```python
from build123d import *

# Parameters (mm, degrees)
ESQUISSE1_W                                  = 200
ESQUISSE1_H                                  = 160
ESQUISSE1_R                                  = 5
ESQUISSE1_R_2                                = 1.75
ESQUISSE1_W_2                                = 10
ESQUISSE1_H_2                                = 10
ESQUISSE1_H_3                                = 30
BOSS_EXTRU_1_DEPTH                           = 5
CONG_2_R                                     = 1
ENL_V_MAT_EXTRU_1_DEPTH                      = 129.16005618
ESQUISSE3_R                                  = 1.75
TROU_CUVE_DIRECTION_DEPTH                    = 129.16005618
ESQUISSE4_R                                  = 1.7
ESQUISSE4_R_2                                = 5
POINTE_AVANT_TROUS_BATTERIES_ET_CABLES_DEPTH = 129.16005618


with BuildPart() as part:
    # Esquisse1 → Boss.-Extru.1 (new body)
    with BuildSketch(Plane(origin=(0, 0, 0), x_dir=(0, 1, 0), z_dir=(0, 0, 1))):
        Rectangle(ESQUISSE1_W, ESQUISSE1_H)
        with Locations(Location((-75, 0, 0), (0, 0, 270))):
            Circle(ESQUISSE1_R, mode=Mode.SUBTRACT)
        with Locations(Location((-57.5, 35.5, 0), (0, 0, 270))):
            Circle(ESQUISSE1_R_2, mode=Mode.SUBTRACT)
        with Locations(Location((-57.5, -35.5, 0), (0, 0, 90))):
            Circle(ESQUISSE1_R_2, mode=Mode.SUBTRACT)
        with Locations(Location((65, 45, 0), (0, 0, 270))):
            Circle(ESQUISSE1_R_2, mode=Mode.SUBTRACT)
        with Locations(Location((65, -45, 0), (0, 0, 90))):
            Circle(ESQUISSE1_R_2, mode=Mode.SUBTRACT)
        with Locations(Location((-31, 37.5, 0), (0, 0, 270))):
            Circle(ESQUISSE1_R_2, mode=Mode.SUBTRACT)
        with Locations(Location((-31, 75, 0), (0, 0, 270))):
            Circle(ESQUISSE1_R_2, mode=Mode.SUBTRACT)
        with Locations(Location((6.5, 75, 0), (0, 0, 270))):
            Circle(ESQUISSE1_R_2, mode=Mode.SUBTRACT)
        with Locations(Location((6.5, 37.5, 0), (0, 0, 270))):
            Circle(ESQUISSE1_R_2, mode=Mode.SUBTRACT)
        with Locations(Location((-31, -46.541307377, 0), (0, 0, 270))):
            Circle(ESQUISSE1_R_2, mode=Mode.SUBTRACT)
        with Locations(Location((-31, -70.091307377, 0), (0, 0, 270))):
            Circle(ESQUISSE1_R_2, mode=Mode.SUBTRACT)
        with Locations(Location((15.5, -46.541307377, 0), (0, 0, 270))):
            Circle(ESQUISSE1_R_2, mode=Mode.SUBTRACT)
        with Locations(Location((15.5, -70.091307377, 0), (0, 0, 270))):
            Circle(ESQUISSE1_R_2, mode=Mode.SUBTRACT)
        with Locations(Location((-4.999283545, 0, 0), (0, 0, 270))):
            Circle(ESQUISSE1_R_2, mode=Mode.SUBTRACT)
        with Locations(Location((85, 33, 0), (0, 0, 270))):
            Circle(ESQUISSE1_R_2, mode=Mode.SUBTRACT)
        with Locations(Location((85.001189598, -32.999999989, 0), (0, 0, 270))):
            Circle(ESQUISSE1_R_2, mode=Mode.SUBTRACT)
        with Locations(Location((19, 33, 0), (0, 0, 270))):
            Circle(ESQUISSE1_R_2, mode=Mode.SUBTRACT)
        with Locations(Location((19.001189598, -32.999999989, 0), (0, 0, 270))):
            Circle(ESQUISSE1_R_2, mode=Mode.SUBTRACT)
        with Locations((-46, 35)):
            Rectangle(ESQUISSE1_W_2, ESQUISSE1_H_2, mode=Mode.SUBTRACT)
        with Locations((7, 0)):
            Rectangle(ESQUISSE1_W_2, ESQUISSE1_H_3, mode=Mode.SUBTRACT)
    extrude(amount=BOSS_EXTRU_1_DEPTH)

    # Congé2
    cong_2_edges = [part.edges().sort_by_distance(p)[0] for p in [
        (-40, -51, 2.5),
        (-30, -51, 2.5),
        (-30, -41, 2.5),
        (-40, -41, 2.5),
        (-15, 2, 2.5),
        (15, 2, 2.5),
        (15, 12, 2.5),
        (-15, 12, 2.5),
    ]]
    fillet(cong_2_edges, radius=CONG_2_R)

    # Esquisse2 → Enlèv. mat.-Extru.1 (cut, through all)
    with BuildSketch(Plane.XY.offset(5)):
        Polygon((-573.580399643, 598.167108478), (-698.698151963, -488.082468479), (684.299979338, -647.380682556), (762.904681953, 702.431902078), align=None)
        Polygon((-110, 40), (0, 160), (110, 40), (110, -40), (0, -160), (-110, -40), align=None, mode=Mode.SUBTRACT)
    extrude(amount=-ENL_V_MAT_EXTRU_1_DEPTH, mode=Mode.SUBTRACT)

    # Esquisse3 → Trou cuve direction (cut, through all)
    with BuildSketch(Plane(origin=(0, 0, 0), x_dir=(0, 1, 0), z_dir=(0, 0, 1))):
        with Locations(Location((-94.001515359, 0.004041019, 0), (0, 0, 270))):
            Circle(ESQUISSE3_R)
    extrude(amount=TROU_CUVE_DIRECTION_DEPTH, mode=Mode.SUBTRACT)

    # Esquisse4 → Pointe avant, trous batteries et cables (cut, through all)
    with BuildSketch(Plane.XY.offset(5)):
        with Locations((-50.974041019, -81.261515359)):
            Circle(ESQUISSE4_R)
        with Locations((-74.974041019, 23.238484641)):
            Circle(ESQUISSE4_R)
        with Locations((50.965958981, -81.261515359)):
            Circle(ESQUISSE4_R)
        with Locations((74.965958981, 23.238484641)):
            Circle(ESQUISSE4_R)
        with Locations((-62.974041019, 33.738484641)):
            Circle(ESQUISSE4_R_2)
        with Locations((62.965958981, 33.738484641)):
            Circle(ESQUISSE4_R_2)
        with Locations((-24.724041019, -20.261515359)):
            Circle(ESQUISSE4_R_2)
        with Locations((24.675958981, -20.261515359)):
            Circle(ESQUISSE4_R_2)
        Polygon((-82.024041019, 47.038484641), (-45.024041019, 103.038484641), (-83.024041019, 103.038484641), (-83.024041019, 47.038484641), align=None)
        Polygon((82.015958981, 47.038484641), (45.015958981, 103.038484641), (83.015958981, 103.038484641), (83.015958981, 47.038484641), align=None)
    extrude(amount=-POINTE_AVANT_TROUS_BATTERIES_ET_CABLES_DEPTH, mode=Mode.SUBTRACT)


solid = part.part
```
Can you work these out from the model? Positions are in its coordinate system, mm. A direction names the side the tool comes from. Coordinates: 2 decimals unless noted, no trailing zeros. Order: outer loops, then holes, each group sorted by start corner. A loop starts at its lowest first (then second) coordinate and runs counter-clockwise, first axis right, second up.
1. If we section it at B-B (y = 36): Please give me the cut outline in (x, z), then the cut area to 3 significant figures.
2. If we section it at D-D (y = 70): Please give me the cut outline in (x, z), then the cut area to 3 significant figures.
3. Thinking about a two-plate mould opening in Y: for faces 1 (the face through (-15, 7, 2)), 2 (the face through (-67.325, -86.555, 2.535)), 3 (the face through (63.74, 74.7, 2.54)), 4 (the face through (-1, -1, 5)), which applies, +Y half, -Y half, draft (parallel to the pull), parting line (faces both ways), or undercut?
4. I'm going to push a flat-ended pin straight in: pin 1 (2 mm diameter, centred on x = 58.5, z = 4, fed in from -Y). Where does the tip first touch, or does it pass through?
5. If we section it at A-A (x = 63.5): Please give me the cut outline in (y, z).
6. I need wall thicknesses on line 1 (Y direction, x = -37.5, z = 2); line 2 (Y direction, x = -7, z = 3.25); line 3 (Y direction, x = -1, z = 3). Which ranges of each line are inside material? Lowest first, please.
7. For faces 5 (the face through (-35, -51, 2)), 6 (the face through (-80, -12, 2)), which set-ups out of +Z, -Z, +X, -X, +Y, -Y let a thin tool reach every point of the face, with its end or its side?
8. If we section it at C-C (z = 1.9): Give the number of separate pieces and of enclosed holes in the cut face, then the cut area to 3 significant figures.
Entries:
1. outline: (-80, 0) - (-67.43, 0) - (-67.43, 5) - (-80, 5) - close; (-58.51, 0) - (58.51, 0) - (58.51, 5) - (-58.51, 5) - close; (67.43, 0) - (80, 0) - (80, 5) - (67.43, 5) - close
1. area: 711 mm2
2. outline: (-66.85, 0) - (66.84, 0) - (66.84, 5) - (-66.85, 5) - close
2. area: 668 mm2
3. face 1: undercut
3. face 2: -Y half
3. face 3: +Y half
3. face 4: draft
4. pin 1: stops at y = -97.27
5. outline: (-90.73, 0) - (28.77, 0) - (28.77, 5) - (-90.73, 5) - close; (38.71, 0) - (75.06, 0) - (75.06, 5) - (38.71, 5) - close
6. line 1: y = -100 to -51, -41 to -32.75, -29.25 to 4.75, 8.25 to 100
6. line 2: y = -100 to 2, 12 to 100
6. line 3: y = -100 to -95.44, -92.56 to -79.9, -70.1 to -6.44, -3.56 to 2, 12 to 100
7. face 5: +Z, -Z
7. face 6: +Z, -Z, -X, +Y, -Y
8. separate pieces: 1
8. enclosed holes: 29
8. area: 28,700 mm2
